Source: three-view drawing plus pictorial views. Frame: mm from the lowest corner of the part. Give positions to 0.01 mm unless a question says otherwise; leave off trailing zeros. Loops run counter-clockwise (first coordinate to the right, second up) from the corner with the lowest first, then second, coordinate; pieces in that order, holes last. Notation, with made-up numbers: (87.25, 39.25) -> (142.25, 39.25) arc R29 cw to (142.25, 67.25) -> close; hole circle Ø11 at (6, 8.5). An arc over 180 degrees is marked (long way). Answer in a Markdown table with one row per item. Add a question column.
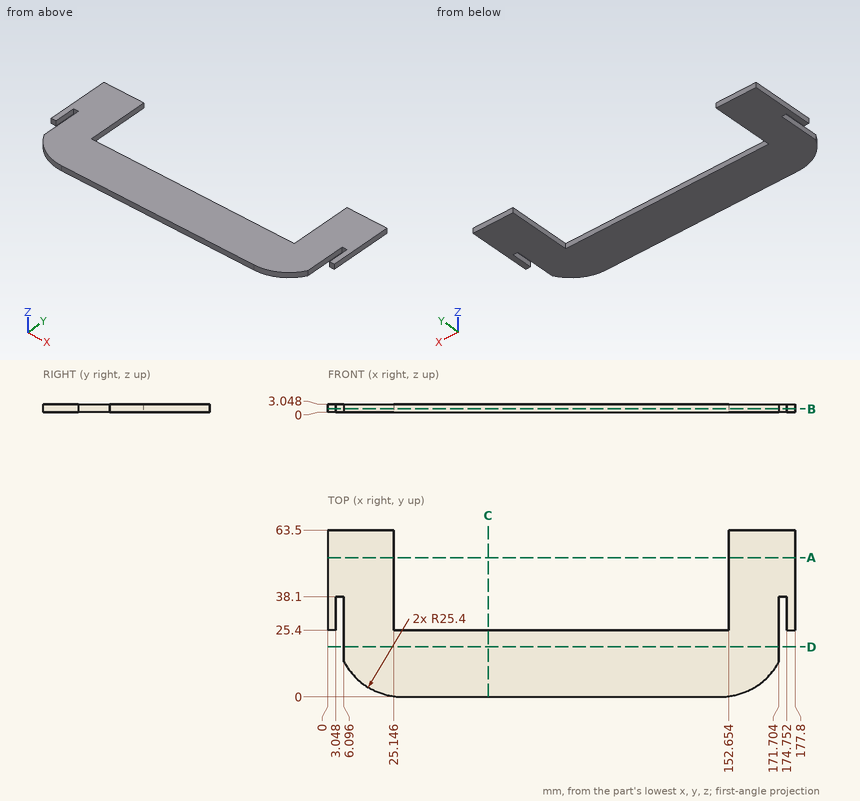
(1) Cut plane A-A on y = 53. Return the cut outline in (x, z).
(2) Cut plane B-B on z = 1.15. Return the cut outline in (x, y).
(3) Cut plane D-D on y = 19. Return the cut outline in (x, z).
(4) Cut plane C-C on x = 61. Return the cut outline in (y, z).
(5) Pin query (flat end, axial travel): pin 1 Ø1 at (x, z) = (40, 2.5) entering from +Y. Return the tip coordinate at first contact, or that it passes through.
(6) Material intervals for line 1 along X through (y, z) = (29.5, 1.7); line 2 along X through (y, z) = (39, 2.05); line 3 along Y through (x, z) = (137, 0.85), sorted ascending. Write a range as from..to.
Answer list:
| question | item | result |
|---|---|---|
| 1 | outline | (0, 0) -> (25.15, 0) -> (25.15, 3.05) -> (0, 3.05) -> close; (152.65, 0) -> (177.8, 0) -> (177.8, 3.05) -> (152.65, 3.05) -> close |
| 2 | outline | (0, 25.4) -> (3.05, 25.4) -> (3.05, 38.1) -> (6.1, 38.1) -> (6.1, 13.34) arc R25.4 ccw to (28.45, 0) -> (149.35, 0) arc R25.4 ccw to (171.7, 13.34) -> (171.7, 38.1) -> (174.75, 38.1) -> (174.75, 25.4) -> (177.8, 25.4) -> (177.8, 63.5) -> (152.65, 63.5) -> (152.65, 25.4) -> (25.15, 25.4) -> (25.15, 63.5) -> (0, 63.5) -> close |
| 3 | outline | (6.1, 0) -> (171.7, 0) -> (171.7, 3.05) -> (6.1, 3.05) -> close |
| 4 | outline | (0, 0) -> (25.4, 0) -> (25.4, 3.05) -> (0, 3.05) -> close |
| 5 | pin 1 | stops at y = 25.4 |
| 6 | line 1 | x = 0..3.05, 6.1..25.15, 152.65..171.7, 174.75..177.8 |
| 6 | line 2 | x = 0..25.15, 152.65..177.8 |
| 6 | line 3 | y = 0..25.4 |
